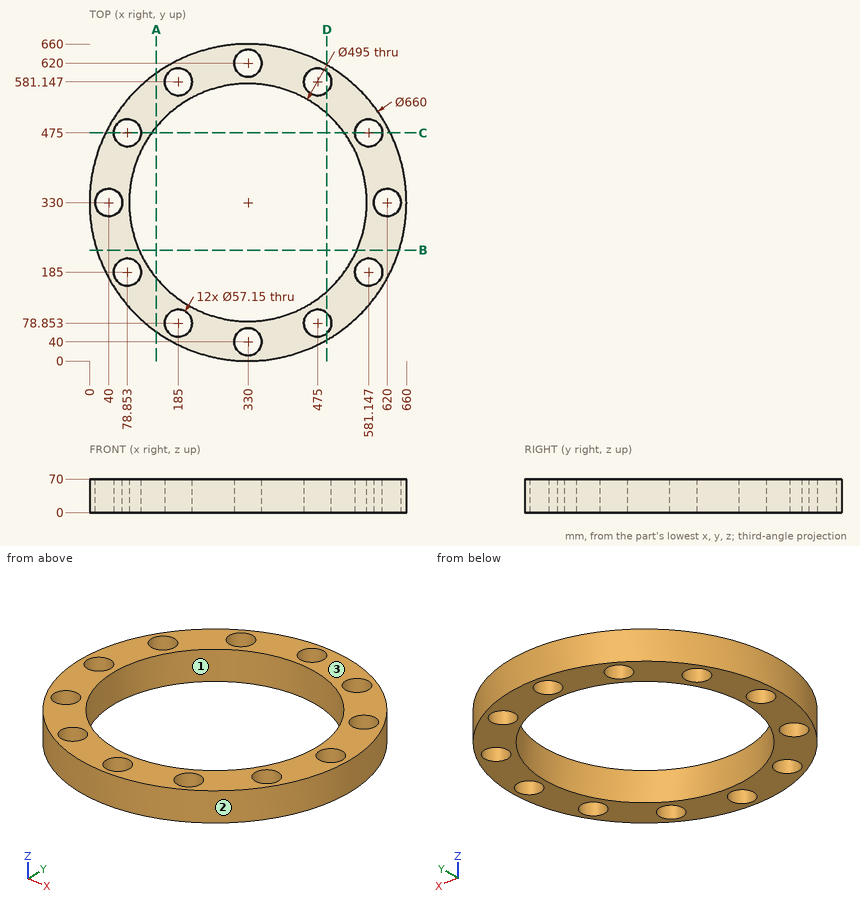
Study the drawing (mm; zero at the part's minimum x, y, z) and answer. Coordinates: 2 decimals unless noted, no trailing zeros. Loops run counter-clockwise (first coordinate to the right, second up) from the corner with the lowest first, then second, coordinate; pieces in that order, holes last. Notation, with made-up numbers: (33.5, -22) -> (92.5, -22) arc R29 cw to (92.5, 14) -> close; hole circle Ø2 at (-21.5, -29). An arc over 180 degrees is marked (long way). Answer in a Markdown table with one row per item. Add a question column.
1. The part is cut by section A-A, the plane x = 139. Write down the section's boundary in (y, z).
2. The part is cut by section C-C, the plane y = 475. Write down the section's boundary in (x, z).
3. The part is cut by section D-D, the plane x = 494. Write down the section's boundary in (y, z) (1 decimal), then the cut area to 3 significant figures.
4. The part is cut by section B-B, the plane y = 231. Write down the section's boundary in (x, z), then the cut area to 3 significant figures.
5. Determine the mould class of the marked faces 1, 2 and 3 for opening direction X: +X half, -X half, draft (parallel to the pull), parting line (faces both ways), or undercut.
6. Flat-ended cylindrical pins translate along their axes: P1, Ø5, axis at x = 252, z = 54.5, coming from the +Y side; P2, Ø6, axis at x = 104.5, z = 40.5, coming from the +Y side; P3, Ø5, axis at y = 570, z = 18, coming from the -X side (1 decimal). Find the tip coordinate at first contact, or state that the pin passes through.
7. Consider line 1 (Y direction, x = 330, z = 48) (1 decimal); line 2 (Y direction, x = 475, z = 37); line 3 (X direction, y = 492.5, z = 48.5) (1 decimal). Determine where each line is inside the solid, lowest interval first. Write a range as [from, to].
Answer below:
| question | item | result |
|---|---|---|
| 1 | outline | (60.89, 0) -> (172.6, 0) -> (172.6, 70) -> (60.89, 70) -> close; (487.4, 0) -> (599.11, 0) -> (599.11, 70) -> (487.4, 70) -> close |
| 2 | outline | (33.56, 0) -> (50.28, 0) -> (50.28, 70) -> (33.56, 70) -> close; (107.43, 0) -> (129.42, 0) -> (129.42, 70) -> (107.43, 70) -> close; (530.58, 0) -> (552.57, 0) -> (552.57, 70) -> (530.58, 70) -> close; (609.72, 0) -> (626.44, 0) -> (626.44, 70) -> (609.72, 70) -> close |
| 3 | outline | (43.6, 0) -> (57.5, 0) -> (57.5, 70) -> (43.6, 70) -> close; (100.2, 0) -> (144.6, 0) -> (144.6, 70) -> (100.2, 70) -> close; (515.4, 0) -> (559.8, 0) -> (559.8, 70) -> (515.4, 70) -> close; (602.5, 0) -> (616.4, 0) -> (616.4, 70) -> (602.5, 70) -> close |
| 3 | area | 8,160 mm2 |
| 4 | outline | (15.2, 0) -> (103.16, 0) -> (103.16, 70) -> (15.2, 70) -> close; (556.84, 0) -> (644.8, 0) -> (644.8, 70) -> (556.84, 70) -> close |
| 4 | area | 12,300 mm2 |
| 5 | face 1 | undercut |
| 5 | face 2 | parting line |
| 5 | face 3 | draft |
| 6 | P1 | y = 651.25 |
| 6 | P2 | y = 573.71 |
| 6 | P3 | x = 100.9 |
| 7 | line 1 | [0, 11.4], [68.6, 82.5], [577.5, 591.4], [648.6, 660] |
| 7 | line 2 | [33.56, 50.28], [107.43, 129.42], [530.58, 552.57], [609.72, 626.44] |
| 7 | line 3 | [42.8, 56.3], [101.4, 143.3], [516.7, 558.6], [603.7, 617.2] |
